Geometry: see drawing. Coordinates: mm, zero at the bounding-box minimum. A direction names the side the tool comes from. Round coordinates to 2 decimals unless told otherwise and drop trailing zeros. Loops run counter-clockwise (first coordinate to the right, second up) from the corner with the lowest first, then second, coordinate; pieces in that order, holes last.
(1) Cut plane C-C, the plane z = 21.5. Output: boundary loops of the cut face in (x, y) (3 decimals), and give its area (3 significant figures).
(2) Line query: line 1 (Y direction, x = 6.35, z = 1.05) (3 decimals); line 2 (X direction, y = 114, z = 1); line 3 (Y direction, x = 11.25, z = 26.5) (3 decimals). Output: solid intervals per line, ascending.
(3) First-contact query: pin 1 Ø5.5 at (x, y) = (6.35, 114.3) entering from +Z; pin 2 Ø1 at (x, z) = (3.5, 10) entering from -Y; pin 3 Ø3 at (x, z) = (8.5, 15) entering from +Y (3 decimals). Flat tips, straight axial feed; report the tip coordinate or a pass-through.
(4) Access query for the marked faces 1, 2 and 3. Directions: +Z, -Z, +X, -X, +Y, -Y. A direction counts if a zero-diameter tool reaches every point of the face in a straight line with its end or side. Return the directions, or none.
(5) Cut plane A-A, the plane y = 114.3. Output: boundary loops of the cut face in (x, z) (3 decimals), and give its area (3 significant figures).
(6) Draft query along Z for the marked faces 4, 5 and 6. Return one class per face: released by +Z, released by -Z, zero draft, split by the parting line, or undercut.
(7) Cut plane D-D, the plane y = 47. Output: boundary loops of the cut face in (x, z) (3 decimals), and give its area (3 significant figures).
(8) Cut plane B-B, the plane x = 6.35. Output: boundary loops of the cut face in (y, z) (3 decimals).
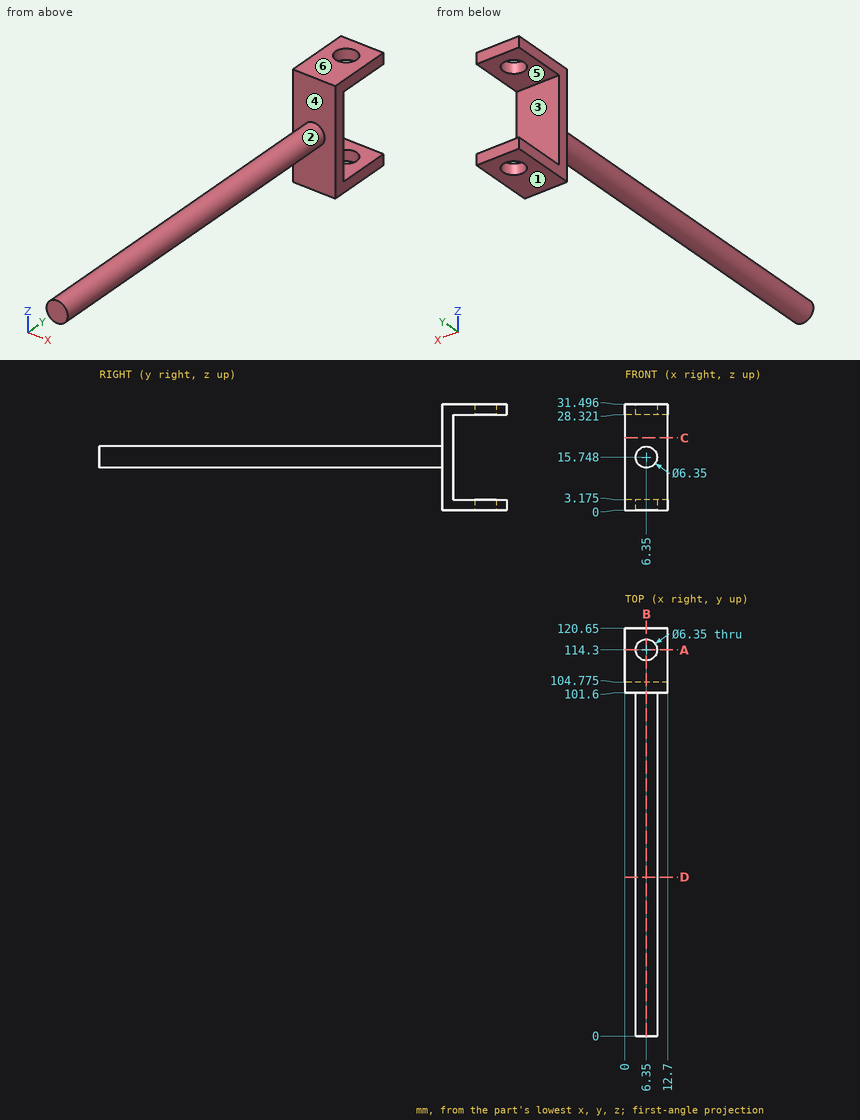
Reported:
1. outline: (0, 101.6) - (12.7, 101.6) - (12.7, 104.775) - (0, 104.775) - close
1. area: 40.3 mm2
2. line 1: y = 101.6 to 111.125, 117.475 to 120.65
2. line 2: x = 0 to 3.19, 9.51 to 12.7
2. line 3: y = 101.6 to 104.775
3. pin 1: passes through
3. pin 2: stops at y = 101.6
3. pin 3: stops at y = 104.775
4. face 1: -Z, +X, -X, +Y, -Y
4. face 2: -Y
4. face 3: +X, -X, +Y
5. outline: (0, 0) - (3.175, 0) - (3.175, 3.175) - (0, 3.175) - close; (0, 28.321) - (3.175, 28.321) - (3.175, 31.496) - (0, 31.496) - close; (9.525, 0) - (12.7, 0) - (12.7, 3.175) - (9.525, 3.175) - close; (9.525, 28.321) - (12.7, 28.321) - (12.7, 31.496) - (9.525, 31.496) - close
5. area: 40.3 mm2
6. face 4: zero draft
6. face 5: undercut
6. face 6: released by +Z
7. outline: circle Ø6.35 at (6.35, 15.748)
7. area: 31.7 mm2
8. outline: (0, 12.573) - (101.6, 12.573) - (101.6, 0) - (111.125, 0) - (111.125, 3.175) - (104.775, 3.175) - (104.775, 28.321) - (111.125, 28.321) - (111.125, 31.496) - (101.6, 31.496) - (101.6, 18.923) - (0, 18.923) - close; (117.475, 0) - (120.65, 0) - (120.65, 3.175) - (117.475, 3.175) - close; (117.475, 28.321) - (120.65, 28.321) - (120.65, 31.496) - (117.475, 31.496) - close
